Source: CAD feature listing. Evaluate the final solid. Frame: model axes, mm. A direction names the side the tool comes from. Give positions to 0.01 mm unless a question says otherwise; leave off trailing zeros. Order: outer loops, then holes, each group sorted by start corner. A loop starts at its lowest first (then second) coordinate and runs counter-clockwise, first axis right, second up. Notation, with made-up numbers: (-15, -13.75) -> (9, -13.75) arc R4 cw to (9, -7.75) -> close; hole circle Ø2 at (-19.75, 78.25). An arc over 180 degrees is marked (long way). Answer in a Markdown table with one row per item.
```python
from build123d import *

# Parameters (mm, degrees)
SZKIC1_W                                             = 35
SZKIC1_H                                             = 100
DODANIE_WYCI_GNI_CIE1_DEPTH                          = 14
SFAZOWANIE1_SIZE                                     = 10
POG_BIENIE_WALCOWE_POD_M6_WKR_T_DO_CZ_CI_D           = 6.5
POG_BIENIE_WALCOWE_POD_M6_WKR_T_DO_CZ_CI_CBORE_D     = 11
POG_BIENIE_WALCOWE_POD_M6_WKR_T_DO_CZ_CI_CBORE_DEPTH = 6
OTW_R_GWINTOWANY_M6X1_01_D                           = 5
OTW_R_GWINTOWANY_M6X1_01_DEPTH                       = 17
OTW_R_GWINTOWANY_M6X1_01_TIP                         = 1.502151548


with BuildPart() as part:
    # Szkic1 → Dodanie-wyciągnięcie1 (new body)
    with BuildSketch(Plane.XY):
        with Locations((17.5, 50)):
            Rectangle(SZKIC1_W, SZKIC1_H)
    extrude(amount=DODANIE_WYCI_GNI_CIE1_DEPTH)

    # Sfazowanie1
    sfazowanie1_edges = [part.edges().sort_by_distance(p)[0] for p in [
        (35, 100, 7),
    ]]
    chamfer(sfazowanie1_edges, length=SFAZOWANIE1_SIZE)

    # Pogłębienie walcowe pod M6 Wkręt do części metalowych z łbem sześciokątnym1 (through all)
    with Locations(Plane(origin=(35, 0, 0), x_dir=(0, 0, -1), z_dir=(1, 0, 0))):
        with Locations((-7, 70), (-7, 25)):
            CounterBoreHole(POG_BIENIE_WALCOWE_POD_M6_WKR_T_DO_CZ_CI_D / 2, POG_BIENIE_WALCOWE_POD_M6_WKR_T_DO_CZ_CI_CBORE_D / 2, POG_BIENIE_WALCOWE_POD_M6_WKR_T_DO_CZ_CI_CBORE_DEPTH)

    # Otwór gwintowany M6x1.01
    with Locations(Plane(origin=(0, 0, 0), x_dir=(-1, 0, 0), z_dir=(0, -1, 0))):
        with Locations((-17.5, -7)):
            Hole(OTW_R_GWINTOWANY_M6X1_01_D / 2, depth=OTW_R_GWINTOWANY_M6X1_01_DEPTH)
            with Locations((0, 0, -(OTW_R_GWINTOWANY_M6X1_01_DEPTH + OTW_R_GWINTOWANY_M6X1_01_TIP / 2))):  # 118° drill point
                Cone(0, OTW_R_GWINTOWANY_M6X1_01_D / 2, OTW_R_GWINTOWANY_M6X1_01_TIP, mode=Mode.SUBTRACT)


solid = part.part
```
(1) Access query for faces 1 (the cylindrical face through (15, 9, 7)), 2 (the cylindrical face through (14.297, 68.022, 4.421)), 3 (the cylindrical face through (32.042, 26.652, 1.754)). Directions: +Z, -Z, +X, -X, +Y, -Y. A direction counts if a zero-diameter tool reaches every point of the face in a straight line with its end or side. Return the directions, or none.
A:
| item | result |
|---|---|
| face 1 | -Y |
| face 2 | +X, -X |
| face 3 | +X |
(2) Pull-direction query (Z, two-part tool) for faces 4 (the cylindrical face through (14.297, 21.827, 6.295)), 5 (the cylindrical face through (32.042, 75.453, 7.716)), 6 (the flat face through (17, 51, 0)), 7 (the flat face through (35, 44, 7)); classes: +Z half, -Z half, draft (parallel to the pull), parting line (faces both ways), or undercut.
A:
| item | result |
|---|---|
| face 4 | undercut |
| face 5 | undercut |
| face 6 | -Z half |
| face 7 | draft |
(3) Ray query, probe 1 along Y at (x, z) = (14.5, 7); probe 2 along Y at (x, z) = (18.5, 7); probe 3 along X at (y, z) = (73, 5.25). Return the intervals inside material, ascending.
A:
| item | result |
|---|---|
| probe 1 | y = 0 to 21.75, 28.25 to 66.75, 73.25 to 100 |
| probe 2 | y = 17.9 to 21.75, 28.25 to 66.75, 73.25 to 100 |
| probe 3 | x = 0 to 29 |
(4) Section query C-C (y = 7.5). Return the cut outline in (x, z), plus the area to 3 significant figures.
A:
| item | result |
|---|---|
| outline | (0, 0) -> (35, 0) -> (35, 14) -> (0, 14) -> close; hole circle Ø5 at (17.5, 7) |
| area | 470 mm^2 |
(5) Section query B-B (x = 12). Return the cut outline in (y, z).
A:
| item | result |
|---|---|
| outline | (0, 0) -> (100, 0) -> (100, 14) -> (0, 14) -> close; hole circle Ø6.5 at (25, 7); hole circle Ø6.5 at (70, 7) |
(6) Section query D-D (x = 30). Return the cut outline in (y, z).
A:
| item | result |
|---|---|
| outline | (0, 0) -> (95, 0) -> (95, 14) -> (0, 14) -> close; hole circle Ø11 at (25, 7); hole circle Ø11 at (70, 7) |
(7) Section query A-A (y = 25). Return the cut outline in (x, z), plus the area to 4 significant figures.
A:
| item | result |
|---|---|
| outline | (0, 0) -> (35, 0) -> (35, 1.5) -> (29, 1.5) -> (29, 3.75) -> (0, 3.75) -> close; (0, 10.25) -> (29, 10.25) -> (29, 12.5) -> (35, 12.5) -> (35, 14) -> (0, 14) -> close |
| area | 235.5 mm^2 |
(8) First-contact query: pin 1 Ø6 at (y, z) = (70, 7) entering from +X. Flat tip, straight axial feed; report the tip coordinate or a pass-through.
A:
| item | result |
|---|---|
| pin 1 | passes through |
